Work out the finished part from the listing and answer in its coordinate system (mm). A direction names the side the tool comes from. Round coordinates to 2 decimals unless told otherwise and drop trailing zeros. Order: outer loops, then holes, each group sorted by start corner. A loop starts at its lowest first (then second) coordinate and runs counter-clockwise, first axis right, second up. Notation, with made-up numbers: (6.25, 54.25) - (43.25, 54.25) arc R12 ccw to (43.25, 74.25) - close; hole circle Ø4 at (53.25, -37.75). An arc over 180 degrees is marked (long way). Use one line per item in the form item = value. Start each with the question number.
Q1. Which of the six approach directions +Z, -Z, +X, -X, +Y, -Y give full straight-line access (tool end or side, diameter ignored) to faces 4 (the flat face through (-0.52, 7.92, -22.65)), 5 (the flat face through (-3, 0, -41)), 6 (the flat face through (11.18, 15.17, -0.26))?
Q2. The part is cut by section C-C on y = 16. Determine the outline of the cut face in (x, z) (3 decimals), plus the area to 3 significant figures.
Q3. Find the intervals of material crossed by line 1 (Z direction, x = 18.95, y = 28); line 2 (X direction, y = 25.5, z = 20); line 3 (X direction, y = 4.5, z = 0), in increasing order. Write a range as [from, to].
Q4. The part is cut by section D-D on x = -34.5. Determine the outline of the cut face in (y, z) (3 decimals), plus the area to 3 significant figures.
Q5. The part is cut by section B-B on z = 25. State how many separate pieces and enclosed holes the cut face has, plus the area to 3 significant figures.
Q6. The part is cut by section A-A on y = 28. Determine the outline of the cut face in (x, z).
Q7. For a pull along Z with two mould halves and no side action, classify faces 1 (the cylindrical face through (18.993, 25.581, -21.206)), 2 (the flat face through (0.555, 8.366, 23.938)), 3 (the flat face through (19.5, 23, 0)) as +Z half, -Z half, draft (parallel to the pull), parting line (faces both ways), or undercut.
Q8. Given P1, Ø6, axis at x = 24.5, y = 21.5, coming from the +Z side; P2, Ø17, axis at y = 12.5, z = -12, coming from the +X side (3 decimals); P3, Ø0.5, axis at x = -19, y = 11.5, coming from the -Z side; P4, Ø17, axis at y = 19.5, z = -9, coming from the -X side, each flat-ended and moving along its own axis, determine where each tip first touches the part or whether it passes through.
from build123d import *

# Parameters (mm, degrees)
F0_W      = 75
F0_H      = 75
F4_T      = 1
F0_W_2    = 85
F0_H_2    = 85
F5_DEPTH  = 1
F7_W      = 1
F7_H      = 70
F9_R      = 4.5
F10_DEPTH = 62.001


# Not quite as in the source:
# - a pattern or mirror of a feature is missing from the dataset's text; its kind, count and spacing are read off the source's solid


with BuildPart() as f3:
    # F0 (on Front) → F3 section 0
    with BuildSketch(Plane.XZ, mode=Mode.PRIVATE) as f3_s0:
        Rectangle(F0_W, F0_H)
    loft([f3_s0.sketch, Vertex(0, 20, 0)])

    # F4
    f4_openings = [f3.faces().sort_by_distance(p)[0] for p in [
        (0, 0, 0),
    ]]
    offset(amount=F4_T, openings=f4_openings, kind=Kind.INTERSECTION)

    # F0 (on Front) → F5 (join)
    with BuildSketch(Plane.XZ):
        Rectangle(F0_W_2, F0_H_2)
        Rectangle(F0_W, F0_H, mode=Mode.SUBTRACT)
    extrude(amount=F5_DEPTH)

    # F7 (on offset) → F8 (join, up to the next surface of F3)
    with BuildSketch(Plane.XZ.offset(-36)):
        with Locations((-19, 0)):
            Rectangle(F7_W, F7_H)
    f8 = extrude(until=Until.NEXT)

    # F8_copies: F8 across plane
    add(f8.mirror(Plane(origin=(0, 0, 0), x_dir=(0, 0, 1), z_dir=(1, 0, 0))))

    # F9 (on face) → F10 (cut, through all)
    with BuildSketch(Plane(origin=(-19.5, 0, 0), x_dir=(0, -1, 0), z_dir=(-1, 0, 0))):
        with Locations((-28, -25)):
            Circle(F9_R)
        with Locations((-28, 25)):
            Circle(F9_R)
    extrude(amount=-F10_DEPTH, mode=Mode.SUBTRACT)


solid = f3.part
Found:
q1.face_4 = -Y
q1.face_5 = +Y
q1.face_6 = +Z, -Z, +Y
q2.outline = (-19.5, -35) - (-18.5, -35) - (-18.5, 35) - (-19.5, 35) - close; (-9.625, -9.625) - (9.625, -9.625) - (9.625, 9.625) - (-9.625, 9.625) - close; (18.5, -35) - (19.5, -35) - (19.5, 35) - (18.5, 35) - close; hole (-7.5, -7.5) - (7.5, -7.5) - (7.5, 7.5) - (-7.5, 7.5) - close
q2.area = 286 mm²
q3.line_1 = [-35, -29.5], [-20.5, 20.5], [29.5, 35]
q3.line_2 = [-19.5, -18.5], [18.5, 19.5]
q3.line_3 = [-31.19, -29.06], [29.06, 31.19]
q4.outline = (-1, -42.5) - (0, -42.5) - (0, -39.625) - (2.733, -34.5) - (2.733, 34.5) - (0, 39.625) - (0, 42.5) - (-1, 42.5) - (-1, 37.5) - (0, 37.5) - (1.6, 34.5) - (1.6, -34.5) - (0, -37.5) - (-1, -37.5) - close
q4.area = 97.4 mm²
q5.separate_pieces = 3
q5.enclosed_holes = 0
q5.area = 136 mm²
q6.outline = (-19.5, -35) - (-18.5, -35) - (-18.5, -29.5) - (-19.5, -29.5) - close; (-19.5, -20.5) - (-18.5, -20.5) - (-18.5, 20.5) - (-19.5, 20.5) - close; (-19.5, 29.5) - (-18.5, 29.5) - (-18.5, 35) - (-19.5, 35) - close; (18.5, -35) - (19.5, -35) - (19.5, -29.5) - (18.5, -29.5) - close; (18.5, -20.5) - (19.5, -20.5) - (19.5, 20.5) - (18.5, 20.5) - close; (18.5, 29.5) - (19.5, 29.5) - (19.5, 35) - (18.5, 35) - close
q7.face_1 = undercut
q7.face_2 = +Z half
q7.face_3 = draft
q8.P1 = through
q8.P2 = 32.125
q8.P3 = -35
q8.P4 = -19.5
